Verification items for the finished model (mm, model axes). Face numbers are marked on the shaded views. A direction names the side the tool comes from. Coordinates: 2 decimals unless noted, no trailing zeros. Order: outer loops, then holes, each group sorted by start corner. A loop starts at its lowest first (then second) coordinate and runs counter-clockwise, first axis right, second up. Notation, with made-up numbers: (-19, 82) -> (1, 82) arc R14 ccw to (1, 108) -> close; hole circle Ø5 at (-12.75, 89.25). An arc over 180 degrees is marked (long way). Write item = value, one per line. Start each with the question number.
1. Cross-section at C-C on z = 93. Record the cut outline in (x, y).
2. Cross-section at B-B on y = 186. Record the cut outline in (x, z).
3. Go/stop test with flat-tipped pins: P1, Ø3, axis at x = -9.5, z = 77.5, coming from the +Y side; P2, Ø10, axis at x = 11.5, y = 192, coming from the -Z side; P3, Ø8, axis at x = 2, z = 91.5, coming from the +Y side. Record where each tip stops, or that it passes through.
4. Thickness scan on line 1 along Z through (x, y) = (5.75, 179); line 2 along Y through (x, z) = (0.25, 64); line 3 along Y through (x, z) = (1.5, 83.5). Record the ranges inside material, lowest first. Write a range as from..to.
5. Cross-section at A-A on x = 0. Record the cut outline in (y, z), plus the area to 3 significant figures.
6. Release check for a two-part mould opening along Z. For the marked faces 1, 2 and 3 record: +Z half, -Z half, draft (parallel to the pull), parting line (faces both ways), or undercut.
7. Set-up check for the marked faces 4 and 5: record each of +Z, -Z, +X, -X, +Y, -Y from which the full face is reachable in a straight line by a thin tool's end or side.
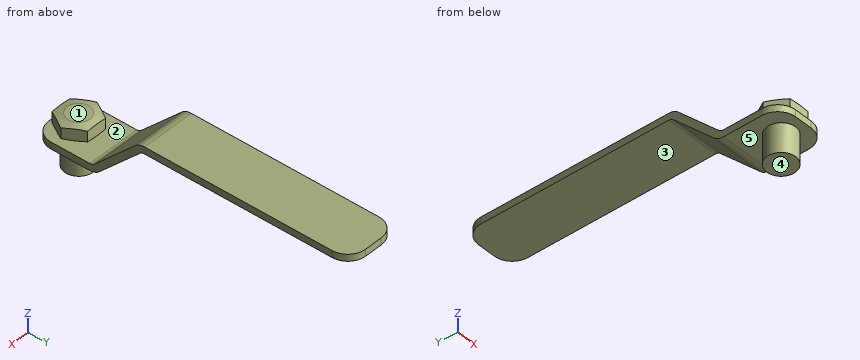
Autodesk Inventor part; units mm, degrees
ref_plane "Work Plane11" through (0, 89, 0) normal (0, -1, 0) x (1, 0, 0)
ref_plane "Work Plane12" through (0, 89, 62.5) normal (0, 0, 1) x (1, 0, 0)
ref_plane "YZ Plane" through (0, 0, 0) normal (1, 0, 0) x (0, 1, 0)
ref_plane "Work Plane11" through (0, 89, 0) normal (0, -1, 0) x (1, 0, 0)
ref_plane "Work Plane12" through (0, 89, 62.5) normal (0, 0, 1) x (1, 0, 0)
sketch "Sketch60" plane through (0, 84.0068, 13.3927) normal (1, 0, 0) x (0, 0, -1)
  line L0 (-59.69, -7.4528) -> (-59.69, 24.2972)
  arc A0 (-59.69, 24.2972) -> (-61.8522, 29.6148) centre (-67.31, 24.2972) ccw
  line L1 (-61.8522, 29.6148) -> (-84.0089, 52.3556)
  arc A1 (-85.09, 55.0144) -> (-84.0089, 52.3556) centre (-81.28, 55.0144) ccw
  line L2 (-85.09, 55.0144) -> (-85.09, 170.3472)
  line L3 (-85.09, 170.3472) -> (-88.9, 170.3472)
  line L4 (-88.9, 170.3472) -> (-88.9, 55.0144)
  arc A2 (-88.9, 55.0144) -> (-86.7378, 49.6968) centre (-81.28, 55.0144) ccw
  line L5 (-86.7378, 49.6968) -> (-64.5811, 26.956)
  arc A3 (-63.5, 24.2972) -> (-64.5811, 26.956) centre (-67.31, 24.2972) ccw
  line L6 (-63.5, 24.2972) -> (-63.5, -7.4528)
  line L7 (-63.5, -7.4528) -> (-59.69, -7.4528)
  line L8 (0, -18.034) -> (0, 124.206)
  line L9 (-28.0662, 4.9932) -> (-56.6073, 4.9932)
  line L10 (-56.6073, -20.0068) -> (-56.6073, 29.9932)
  dimension "d306" = 3.81
  dimension "d307" = 3.81
  dimension "d308" = 3.81
  dimension "d304" = 177.8
  dimension "d311" = 31.75
  dimension "d309" = 31.75
  dimension "d305" = 25.4
  dimension "d310" = 59.69
  dimension "d303" = 12.446
extrude "Extrusion43" add sketch "Sketch60" along normal mid plane 30
fillet "Fillet57" radius 10 4 edges at (-15, 76.554, 74.9877) (15, 76.554, 74.9877) (-15, 254.354, 100.3877) (15, 254.354, 100.3877)
sketch "Sketch61" plane through (-15, 108.304, 76.8927) normal (0, 0, 1) x (1, 0, 0)
  circle A0 centre (15, -19.304) radius 25
  circle A1 centre (15, -19.304) radius 8
  line L0 (3.453, -19.304) -> (9.2265, -9.304)
  line L1 (9.2265, -9.304) -> (20.7735, -9.304)
  line L2 (20.7735, -9.304) -> (26.547, -19.304)
  line L3 (26.547, -19.304) -> (20.7735, -29.304)
  line L4 (20.7735, -29.304) -> (9.2265, -29.304)
  line L5 (9.2265, -29.304) -> (3.453, -19.304)
  dimension "d321" = 16
  dimension "d324" = 20
extrude "Extrusion44" add sketch "Sketch61" against normal blind 20 contours A1
extrude "Extrusion45" add sketch "Sketch61" along normal blind 8 contours A1 | L0 L1 L2 L3 L4 L5
sketch "Sketch62" plane through (0, 0, 0) normal (1, 0, 0) x (0, 1, 0)
  line L0 (89, 76.8927) -> (79, 76.8927)
  line L1 (79, 84.8927) -> (89, 84.8927)
  line L2 (73.6393, 84.8927) -> (73.6393, 82.8927)
  line L3 (73.6393, 82.8927) -> (82.6108, 84.8927)
  line L4 (73.6393, 76.8927) -> (73.6393, 78.8927)
  line L5 (73.6393, 78.8927) -> (82.6108, 76.8927)
  line L6 (89, 115.9127) -> (89, 52.3527)
  line L7 (73.6393, 84.8927) -> (82.6108, 84.8927)
  line L8 (73.6393, 76.8927) -> (82.6108, 76.8927)
  dimension "d330" = 2
revolve "Revolution1" cut sketch "Sketch62" angle 360 about axis through (0, 89, 76.8927) along (0, 0, -1)
equation "\"NB\" = 50"
equation "\"PipeOD\" = 60.325"
equation "\"FlangeOD\" = 165"
equation "\"FlangefaceOD\" = 102"
equation "\"Holedia\" = 19"
equation "\"Holenum\" = 4"
equation "\"PCD\" = 125"
equation "\"Flangethk\" = 16"
equation "\"Flangefacethk\" = 3"
properties part number "Flanged Ball Valve Handle" material "Cast Iron"
Worked out:
q1.outline = (-15, 126.39) -> (15, 126.39) -> (15, 131.84) -> (-15, 131.84) -> close
q2.outline = (-15, 98.48) -> (15, 98.48) -> (15, 102.29) -> (-15, 102.29) -> close
q3.P1 = 117.48
q3.P2 = 98.48
q3.P3 = 134.41
q4.line_1 = 98.48..102.29
q4.line_2 = 81..97
q4.line_3 = 79..99, 116.63..122.09
q5.outline = (76.55, 73.08) -> (81, 73.08) -> (81, 56.89) -> (97, 56.89) -> (97, 73.08) -> (108.3, 73.08) arc R7.62 ccw to (113.62, 75.24) -> (136.36, 97.4) arc R3.81 cw to (139.02, 98.48) -> (254.35, 98.48) -> (254.35, 102.29) -> (139.02, 102.29) arc R7.62 ccw to (133.7, 100.13) -> (110.96, 77.97) arc R3.81 cw to (108.3, 76.89) -> (95.39, 76.89) -> (99, 77.7) -> (99, 84.09) -> (95.39, 84.89) -> (82.61, 84.89) -> (79, 84.09) -> (79, 77.7) -> (82.61, 76.89) -> (76.55, 76.89) -> close
q5.area = 1,130 mm²
q6.face_1 = +Z half
q6.face_2 = undercut
q6.face_3 = -Z half
q7.face_4 = -Z, +X, -X, +Y, -Y
q7.face_5 = -Z
